Check sheet for the drawn part. Datum: minimum x, y, z corner. Units: mm. Coordinates: 2 decimals unless noted, no trailing zeros. Write each loop counter-clockwise with the first axis right and the second up, starting at its lowest first coordinate (ties: lowest second). Pieces come first, ordered by that corner, then holes. Notation, with made-up numbers: (59.5, 2) -> (92.5, 2) arc R31 cw to (92.5, 32) -> close; hole circle Ø4 at (25.25, 39.25). An arc over 180 degrees is marked (long way). Answer in a Markdown table with one row per item. Add a question column.
1. Cross-section at B-B on x = 50. Record the cut outline in (y, z).
2. Cross-section at D-D on x = 92.5. Record the cut outline in (y, z).
3. Scan lines: L1, parallel to Z at x = 50, y = 1.7; L2, parallel to Z at x = 45, y = 0.2. Record each from-to range of solid material in increasing order. Write a range as from..to.
4. Cross-section at A-A on z = 50. Record the cut outline in (x, y).
5. Depth check by flat-ended pin: P1, Ø1.5, axis at x = 88, y = 2, coming from the -Z side; P2, Ø0.9, axis at x = 98.5, y = 1, coming from the +Z side; P3, Ø0.9, axis at y = 2, z = 1, coming from the +X side. Enter the tip coordinate at first touch or a pass-through.
6. Cross-section at C-C on z = 85. Record the cut outline in (x, y).
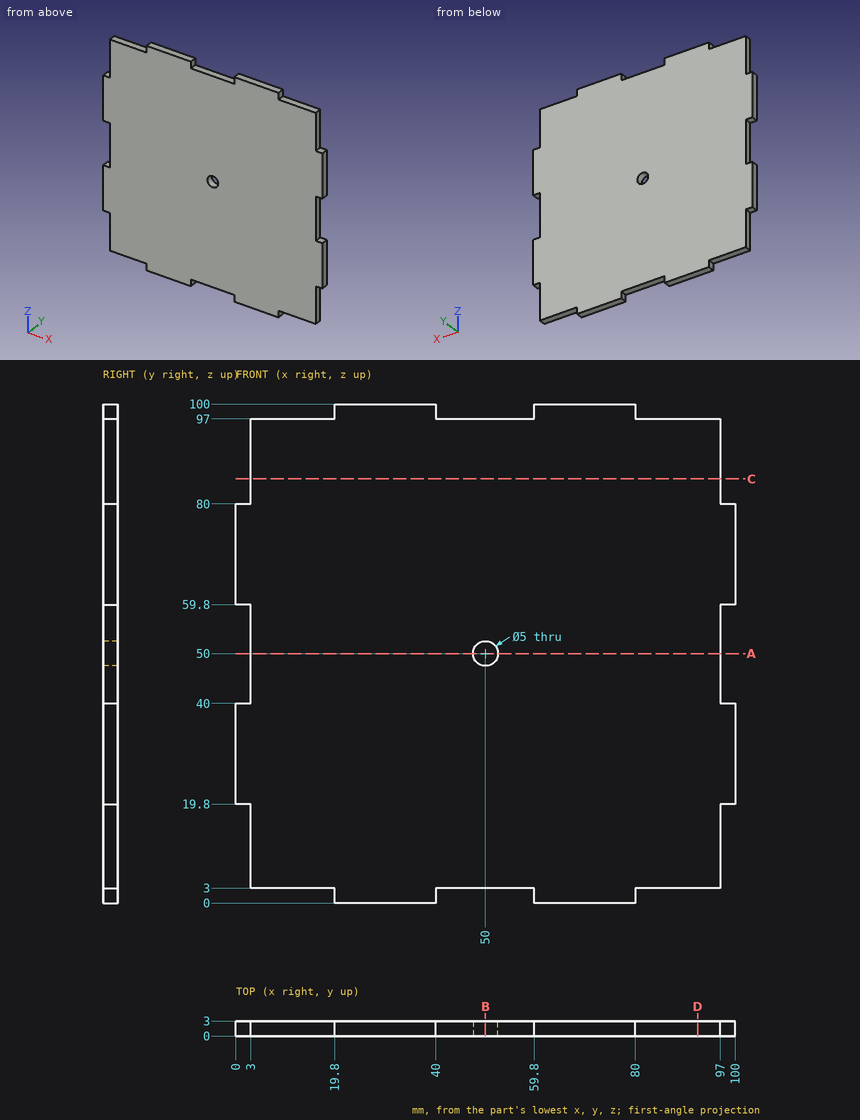
Results found:
| question | item | result |
|---|---|---|
| 1 | outline | (0, 3) -> (3, 3) -> (3, 47.5) -> (0, 47.5) -> close; (0, 52.5) -> (3, 52.5) -> (3, 97) -> (0, 97) -> close |
| 2 | outline | (0, 3) -> (3, 3) -> (3, 97) -> (0, 97) -> close |
| 3 | L1 | z = 3..47.5, 52.5..97 |
| 3 | L2 | z = 3..97 |
| 4 | outline | (3, 0) -> (47.5, 0) -> (47.5, 3) -> (3, 3) -> close; (52.5, 0) -> (97, 0) -> (97, 3) -> (52.5, 3) -> close |
| 5 | P1 | stops at z = 3 |
| 5 | P2 | stops at z = 80 |
| 5 | P3 | stops at x = 80 |
| 6 | outline | (3, 0) -> (97, 0) -> (97, 3) -> (3, 3) -> close |
